Drawing for the job (mm, zero at the part's lowest x, y, z). A direction names the side the tool comes from. Round coordinates to 2 decimals unless told otherwise and drop trailing zeros. Loops run counter-clockwise (first coordinate to the right, second up) from the corner with the lowest first, then second, coordinate; pieces in that order, holes last. Notation, with made-up numbers: (66, 73.25) -> (105, 73.25) arc R20 cw to (105, 109.25) -> close; hole circle Ø11 at (-35, -25.75). An arc over 180 degrees is marked (long way). Put each result on its own line as item: value. Start each with the question number.
Item 1: Cut at A-A, the plane y = 6.5. List the corners of the cut face in (x, z), plus the area to 3 significant figures.
Item 2: Flat gauge pin, fed straight in: pin 1 Ø5 at (x, z) = (22, 39) entering from +Y. Where does the tip first touch, or does it go through?
Item 3: Drill centre lines: probe 1 along X at (y, z) = (1.25, 39); probe 2 along X at (y, z) = (6.5, 10.5); probe 3 along Z at (x, y) = (70, 5.25). Where is each one in solid material? Low to high. Write a range as [from, to].
Item 4: Pull direction X, two halves, no side cores. Call the marked faces 3, 4, 5 and 6: +X half, -X half, draft (parallel to the pull), parting line (faces both ways), or undercut.
Item 5: Cut at D-D, the plane x = 40.5. List the corners of the cut face in (y, z).
Item 6: Cut at B-B, the plane x = 63. List the corners of the cut face in (y, z).
Item 7: Cut at C-C, the plane z = 39. List the corners of the cut face in (x, y), plus the area to 3 significant figures.
Item 8: Tool access for the marked faces 1 and 2: list every direction of +Z, -Z, +X, -X, +Y, -Y with a clear straight run to the whole face (end or side of a thin tool).
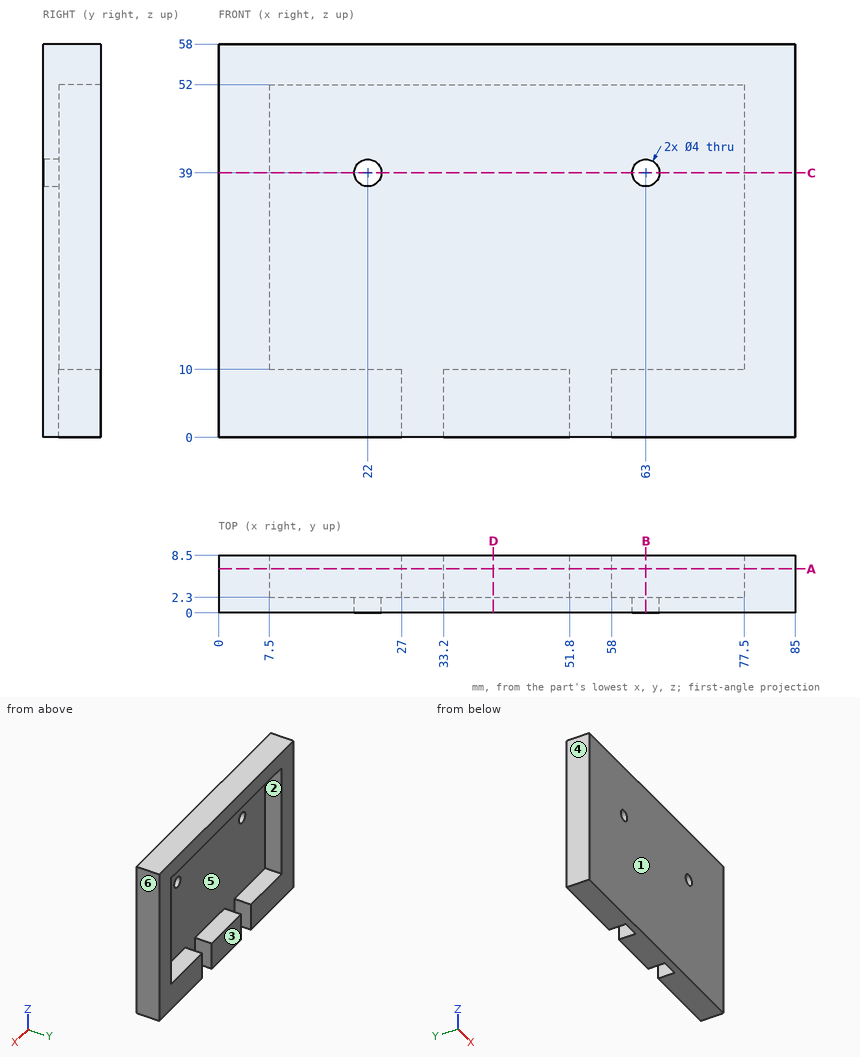
Reply:
1. outline: (0, 0) -> (27, 0) -> (27, 10) -> (7.5, 10) -> (7.5, 52) -> (77.5, 52) -> (77.5, 10) -> (58, 10) -> (58, 0) -> (85, 0) -> (85, 58) -> (0, 58) -> close; (33.2, 0) -> (51.8, 0) -> (51.8, 10) -> (33.2, 10) -> close
1. area: 1,870 mm^2
2. pin 1: stops at y = 2.3
3. probe 1: x = [0, 20], [24, 61], [65, 85]
3. probe 2: x = [0, 7.5], [77.5, 85]
3. probe 3: z = [0, 10], [52, 58]
4. face 3: draft
4. face 4: -X half
4. face 5: undercut
4. face 6: +X half
5. outline: (0, 0) -> (8.5, 0) -> (8.5, 10) -> (2.3, 10) -> (2.3, 52) -> (8.5, 52) -> (8.5, 58) -> (0, 58) -> close
6. outline: (0, 0) -> (8.5, 0) -> (8.5, 10) -> (2.3, 10) -> (2.3, 37) -> (0, 37) -> close; (0, 41) -> (2.3, 41) -> (2.3, 52) -> (8.5, 52) -> (8.5, 58) -> (0, 58) -> close
7. outline: (0, 0) -> (20, 0) -> (20, 2.3) -> (7.5, 2.3) -> (7.5, 8.5) -> (0, 8.5) -> close; (24, 0) -> (61, 0) -> (61, 2.3) -> (24, 2.3) -> close; (65, 0) -> (85, 0) -> (85, 8.5) -> (77.5, 8.5) -> (77.5, 2.3) -> (65, 2.3) -> close
7. area: 270 mm^2
8. face 1: +Z, -Z, +X, -X, -Y
8. face 2: +Y
